```python
from build123d import *

# Parameters (mm, degrees)
CYLINDER065_R          = 1.25
CYLINDER065_DEPTH      = 10
CYLINDER066_R          = 1.25
CYLINDER066_DEPTH      = 10
CYLINDER067_R          = 1.25
CYLINDER067_DEPTH      = 10
CYLINDER068_R          = 1.25
CYLINDER068_DEPTH      = 10
CYLINDER070_R          = 1.25
CYLINDER070_DEPTH      = 10
CYLINDER069_R          = 1.25
CYLINDER069_DEPTH      = 10
CYLINDER063_R          = 1.25
CYLINDER063_DEPTH      = 10
CYLINDER064_R          = 1.25
CYLINDER064_DEPTH      = 10
BOX028_W               = 34
BOX028_H               = 8
BOX028_DEPTH           = 20
BOX029_W               = 34
BOX029_H               = 15
BOX029_DEPTH           = 5
BOX027_W               = 34
BOX027_H               = 15
BOX027_DEPTH           = 5
CUT031_PLACEMENT_ANGLE = 90


with BuildPart() as cylinder065:
    # Cylinder065 → Cylinder065 (new body)
    with BuildSketch(Plane(origin=(87.5, 61, 14), x_dir=(1, 0, 0), z_dir=(0, -1, 0))):
        Circle(CYLINDER065_R)
    extrude(amount=CYLINDER065_DEPTH)


with BuildPart() as cylinder066:
    # Cylinder066 → Cylinder066 (new body)
    with BuildSketch(Plane(origin=(87.5, 11, 14), x_dir=(1, 0, 0), z_dir=(0, -1, 0))):
        Circle(CYLINDER066_R)
    extrude(amount=CYLINDER066_DEPTH)


with BuildPart() as fusion056:
    # Fusion056 base: copy of Cylinder066
    add(cylinder066.part)

    # Fusion056: union Cylinder065
    add(cylinder065.part)


with BuildPart() as fusion056_1:
    # Fusion056 placement: moved
    add(fusion056.part.moved(Location((251.5, 0, 0))))


with BuildPart() as cylinder067:
    # Cylinder067 → Cylinder067 (new body)
    with BuildSketch(Plane(origin=(87.5, 61, 14), x_dir=(1, 0, 0), z_dir=(0, -1, 0))):
        Circle(CYLINDER067_R)
    extrude(amount=CYLINDER067_DEPTH)


with BuildPart() as cylinder068:
    # Cylinder068 → Cylinder068 (new body)
    with BuildSketch(Plane(origin=(87.5, 11, 14), x_dir=(1, 0, 0), z_dir=(0, -1, 0))):
        Circle(CYLINDER068_R)
    extrude(amount=CYLINDER068_DEPTH)


with BuildPart() as fusion057:
    # Fusion057 base: copy of Cylinder068
    add(cylinder068.part)

    # Fusion057: union Cylinder067
    add(cylinder067.part)


with BuildPart() as fusion057_1:
    # Fusion057 placement: moved
    add(fusion057.part.moved(Location((261.5, 0, 0))))


with BuildPart() as cylinder070:
    # Cylinder070 → Cylinder070 (new body)
    with BuildSketch(Plane(origin=(87.5, 61, 14), x_dir=(1, 0, 0), z_dir=(0, -1, 0))):
        Circle(CYLINDER070_R)
    extrude(amount=CYLINDER070_DEPTH)


with BuildPart() as cylinder069:
    # Cylinder069 → Cylinder069 (new body)
    with BuildSketch(Plane(origin=(87.5, 11, 14), x_dir=(1, 0, 0), z_dir=(0, -1, 0))):
        Circle(CYLINDER069_R)
    extrude(amount=CYLINDER069_DEPTH)


with BuildPart() as fusion055:
    # Fusion055 base: copy of Cylinder069
    add(cylinder069.part)

    # Fusion055: union Cylinder070
    add(cylinder070.part)


with BuildPart() as fusion055_1:
    # Fusion055 placement: moved
    add(fusion055.part.moved(Location((270.5, 0, 0))))


with BuildPart() as cylinder063:
    # Cylinder063 → Cylinder063 (new body)
    with BuildSketch(Plane(origin=(87.5, 61, 14), x_dir=(1, 0, 0), z_dir=(0, -1, 0))):
        Circle(CYLINDER063_R)
    extrude(amount=CYLINDER063_DEPTH)


with BuildPart() as cylinder064:
    # Cylinder064 → Cylinder064 (new body)
    with BuildSketch(Plane(origin=(87.5, 11, 14), x_dir=(1, 0, 0), z_dir=(0, -1, 0))):
        Circle(CYLINDER064_R)
    extrude(amount=CYLINDER064_DEPTH)


with BuildPart() as fusion065:
    # Fusion058 base: copy of Cylinder064
    add(cylinder064.part)

    # Fusion058: union Cylinder063
    add(cylinder063.part)


with BuildPart() as fusion065_1:
    # Fusion058 placement: moved
    add(fusion065.part.moved(Location((242.5, 0, 0))))

    # Fusion065: union Fusion056, Fusion057, Fusion055
    add(fusion056_1.part)
    add(fusion057_1.part)
    add(fusion055_1.part)


with BuildPart() as fusion065_2:
    # Fusion065 placement: moved
    add(fusion065_1.part.moved(Location((0, 0, -8))))


with BuildPart() as fusion050:
    # Fusion050 base: copy of Cylinder066
    add(cylinder066.part)

    # Fusion050: union Cylinder065
    add(cylinder065.part)


with BuildPart() as fusion050_1:
    # Fusion050 placement: moved
    add(fusion050.part.moved(Location((251.5, 0, 0))))


with BuildPart() as fusion051:
    # Fusion051 base: copy of Cylinder068
    add(cylinder068.part)

    # Fusion051: union Cylinder067
    add(cylinder067.part)


with BuildPart() as fusion051_1:
    # Fusion051 placement: moved
    add(fusion051.part.moved(Location((261.5, 0, 0))))


with BuildPart() as fusion052:
    # Fusion052 base: copy of Cylinder069
    add(cylinder069.part)

    # Fusion052: union Cylinder070
    add(cylinder070.part)


with BuildPart() as fusion052_1:
    # Fusion052 placement: moved
    add(fusion052.part.moved(Location((270.5, 0, 0))))


with BuildPart() as fusion063:
    # Fusion049 base: copy of Cylinder064
    add(cylinder064.part)

    # Fusion049: union Cylinder063
    add(cylinder063.part)


with BuildPart() as fusion063_1:
    # Fusion049 placement: moved
    add(fusion063.part.moved(Location((242.5, 0, 0))))

    # Fusion064: union Fusion050, Fusion051, Fusion052
    add(fusion050_1.part)
    add(fusion051_1.part)
    add(fusion052_1.part)

    # Fusion063: union Fusion065
    add(fusion065_2.part)


with BuildPart() as fusion063_2:
    # Fusion063 placement: moved
    add(fusion063_1.part.moved(Location((0, -10, 0))))


with BuildPart() as cube007:
    # Box028 → Box028 (new body)
    with BuildSketch(Plane(origin=(0, -10, 0), x_dir=(1, 0, 0), z_dir=(0, 0, 1))):
        with Locations((17, 4)):
            Rectangle(BOX028_W, BOX028_H)
    extrude(amount=BOX028_DEPTH)


with BuildPart() as cube008:
    # Box029 → Box029 (new body)
    with BuildSketch(Plane(origin=(0, -10, 20), x_dir=(1, 0, 0), z_dir=(0, 0, 1))):
        with Locations((17, 7.5)):
            Rectangle(BOX029_W, BOX029_H)
    extrude(amount=BOX029_DEPTH)


with BuildPart() as cut031:
    # Box027 → Box027 (new body)
    with BuildSketch(Plane(origin=(0, -10, -5), x_dir=(1, 0, 0), z_dir=(0, 0, 1))):
        with Locations((17, 7.5)):
            Rectangle(BOX027_W, BOX027_H)
    extrude(amount=BOX027_DEPTH)

    # Fusion067: union Cube007, Cube008
    add(cube007.part)
    add(cube008.part)


with BuildPart() as cut031_1:
    # Fusion067 placement: moved
    add(cut031.part.moved(Location((327, 2, 0))))

    # Cut031: cut Fusion063
    add(fusion063_2.part, mode=Mode.SUBTRACT)


with BuildPart() as cut031_2:
    # Cut031 placement: moved
    add(cut031_1.part.moved(Location((0, -10, 0))).rotate(Axis((0, -10, 0), (1, 0, 0)), CUT031_PLACEMENT_ANGLE))


solid = cut031_2.part
```
Model file for the job. Use its own axes, mm. A direction names the side the tool comes from. Coordinates: 2 decimals unless noted, no trailing zeros. Write each loop counter-clockwise with the first axis right and the second up, starting at its lowest first coordinate (ties: lowest second). Pieces come first, ordered by that corner, then holes. Notation, with made-up numbers: (62, 36) - (97, 36) arc R26 cw to (97, 66) - close; hole circle Ø11 at (41.25, -24.75). An arc over 180 degrees is marked (long way). One line per item, written item: value. Start each with the question number.
1. Slice it at D-D (z = -4). Count the separate pieces of the cut face and the enclosed holes in it, plus the area to 3 significant figures.
2. Tool access for faces 5 (the flat face through (344, -20, 0)), 6 (the cylindrical face through (340.155, -15.521, -3.944)): list every direction of +Z, -Z, +X, -X, +Y, -Y with a clear straight run to the whole face (end or side of a thin tool).
3. Flat gauge pins, fed straight in: pin 1 (4 mm diameter, centred on x = 358, y = -24, fed in from -Z); pin 2 (5 mm diameter, centred on x = 349, y = -18, fed in from +Z); pin 3 (2 mm diameter, centred on x = 349, y = -16, fed in from +Z). Where does each tip first touch, or does it go through?
4. Mould opens along Y. For faces 1 (the cylindrical face through (350.155, -15.521, -3.944)), 2 (the flat face through (327, -20, -2)), 3 (the flat face through (344, -5, 0)), 4 (the cylindrical face through (340.155, -23.521, -3.944)) say: released by +Y, released by -Y, zero draft, split by the parting line, or undercut.
5. Slice it at C-C (y = -16). Write the cut outline in (x, z).
6. Slice it at A-A (z = 3.5). Write the cut outline in (x, y), plus the area to 3 significant figures.
7. Probe line 1 (Y direction, x = 349, z = -4.5); line 2 (Y direction, x = 332.5, z = 0.25); line 3 (Z direction, x = 347, y = -17.5). List the from-to ranges inside material, lowest first. Write a range as from..to.
8. Slice it at B-B (x = 330). Write the cut outline in (y, z).
Answers below:
1. separate pieces: 1
1. enclosed holes: 8
1. area: 981 mm^2
2. face 5: +Z, +X, -X
2. face 6: +Z, -Z
3. pin 1: stops at z = -8
3. pin 2: stops at z = 0
3. pin 3: passes through
4. face 1: undercut
4. face 2: zero draft
4. face 3: released by +Y
4. face 4: undercut
5. outline: (327, -8) - (328.75, -8) - (328.75, 0) - (327, 0) - close; (331.25, -8) - (337.75, -8) - (337.75, 0) - (331.25, 0) - close; (340.25, -8) - (347.75, -8) - (347.75, 0) - (340.25, 0) - close; (350.25, -8) - (356.75, -8) - (356.75, 0) - (350.25, 0) - close; (359.25, -8) - (361, -8) - (361, 0) - (359.25, 0) - close
6. outline: (327, -35) - (361, -35) - (361, -30) - (327, -30) - close; (327, -10) - (361, -10) - (361, -5) - (327, -5) - close
6. area: 340 mm^2
7. line 1: y = -35..-25.25, -22.75..-17.25, -14.75..-5
7. line 2: y = -35..-30, -10..-5
7. line 3: z = -8..0
8. outline: (-35, -8) - (-25.25, -8) - (-25.25, 0) - (-30, 0) - (-30, 7) - (-35, 7) - close; (-22.75, -8) - (-17.25, -8) - (-17.25, 0) - (-22.75, 0) - close; (-14.75, -8) - (-5, -8) - (-5, 7) - (-10, 7) - (-10, 0) - (-14.75, 0) - close
